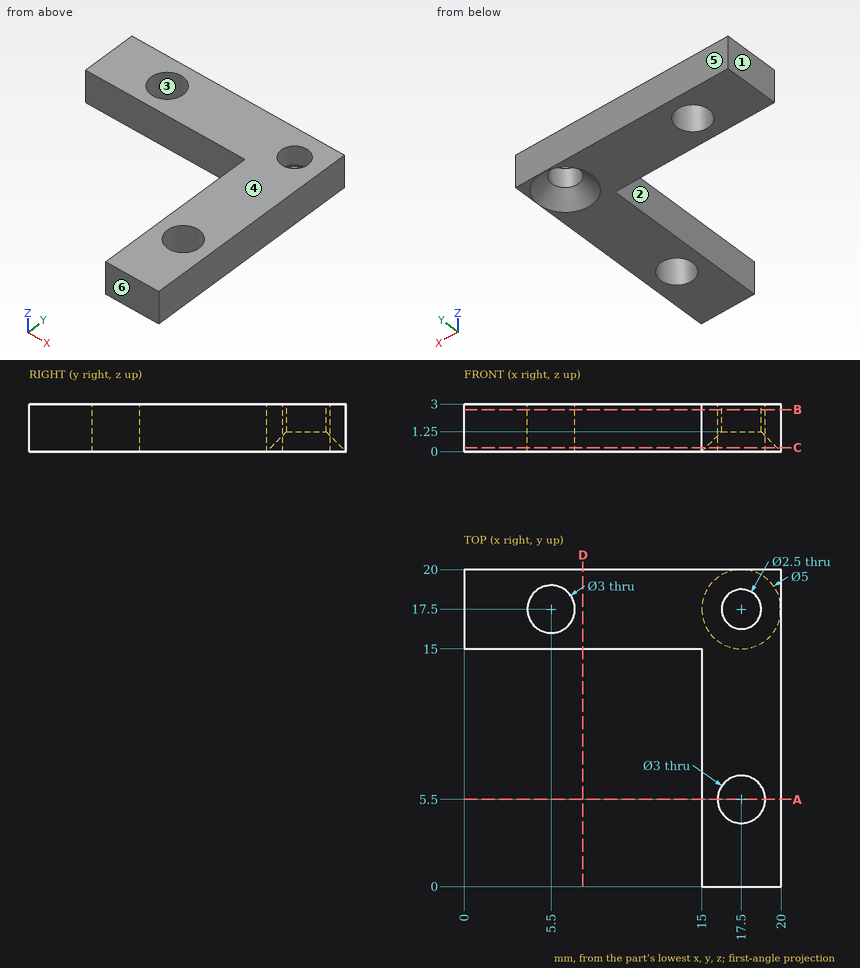
For this review, use the dimensioned drawing (mm, ordinates from the lowest corner) and the shaded views. A direction names the side the tool comes from. Round coordinates to 2 decimals unless told otherwise and drop trailing zeros. Order: outer loops, then holes, each group sorted by start corner. A loop starts at its lowest first (then second) coordinate and runs counter-clockwise, first axis right, second up. Notation, with made-up numbers: (-12.5, -9.75) -> (21.5, -9.75) arc R18 cw to (21.5, 5.25) -> close; hole circle Ø1 at (50, 14.25). An arc over 180 degrees is marked (long way). Write item = value, one per line. Start each with the question number.
Item 1: Consider section B-B on z = 2.65. Write out the cut boundary in (x, y).
Item 2: Consider section C-C on z = 0.25. Write out the cut boundary in (x, y).
Item 3: Consider section A-A on y = 5.5. Write out the cut boundary in (x, z), plus the area to 3 significant figures.
Item 4: For the marked faces 1 and 2, list the 3-axis set-ups (+Z, -Z, +X, -X, +Y, -Y) from which the entire face can be reached by the end or side of a thin tool; tool diameter is ignored.
Item 5: Clearance check with flat-ended pins moving along their axes: pin 1 Ø1.5 at (y, z) = (11, 2) entering from -X; pin 2 Ø4 at (x, y) = (5.5, 17.5) entering from +Z; pin 3 Ø2 at (x, y) = (17.5, 17.5) entering from +Z; pin 4 Ø1.5 at (x, z) = (7, 1) entering from -Y. State where each tip first meets the part, or that it passes through.
Item 6: Consider section D-D on x = 7.5. Write out the cut boundary in (y, z).
Item 7: Mouldability with a two-part tool opening along Y and no side actions: class the marked faces 3, 4, 5 and 6 as released by +Y, released by -Y, zero draft, split by the parting line, or undercut.
Item 8: For line 1 along Y through (x, z) = (17.5, 1.8); line 2 along Y through (x, z) = (5.5, 1.65), list the stretches that pass through material, from the lowest coordinate up.
Conclusion:
q1.outline = (0, 15) -> (15, 15) -> (15, 0) -> (20, 0) -> (20, 20) -> (0, 20) -> close; hole circle Ø3 at (5.5, 17.5); hole circle Ø3 at (17.5, 5.5); hole circle Ø2.5 at (17.5, 17.5)
q2.outline = (0, 15) -> (15, 15) -> (15, 0) -> (20, 0) -> (20, 20) -> (0, 20) -> close; hole circle Ø3 at (5.5, 17.5); hole circle Ø4.5 at (17.5, 17.5); hole circle Ø3 at (17.5, 5.5)
q3.outline = (15, 0) -> (16, 0) -> (16, 3) -> (15, 3) -> close; (19, 0) -> (20, 0) -> (20, 3) -> (19, 3) -> close
q3.area = 6.00 mm2
q4.face_1 = +Z, -Z, -X, +Y, -Y
q4.face_2 = +Z, -Z, -X, -Y
q5.pin_1 = 15
q5.pin_2 = 3
q5.pin_3 = through
q5.pin_4 = 15
q6.outline = (15, 0) -> (20, 0) -> (20, 3) -> (15, 3) -> close
q7.face_3 = undercut
q7.face_4 = zero draft
q7.face_5 = released by +Y
q7.face_6 = released by -Y
q8.line_1 = 0 to 4, 7 to 16.25, 18.75 to 20
q8.line_2 = 15 to 16, 19 to 20
